Check sheet for the modelled part. Datum: model origin and axes. Units: mm. Round coordinates to 2 decimals unless told otherwise and drop trailing zeros. Order: outer loops, then holes, each group sorted by start corner. A loop starts at its lowest first (then second) coordinate and runs counter-clockwise, first axis right, second up.
(1) Thickness scan on probe 1 along Y at (x, z) = (24, 1.5); probe 2 along Y at (x, z) = (58, 4.25); probe 3 along Y at (x, z) = (66, 7.5). Record the ranges inside material, lowest first.
(2) Sectioned sample at A-A, the plane x = 42.5. Enter the section's corners in (y, z).
(3) Sectioned sample at C-C, the plane y = 44.5. Enter the section's corners in (x, z).
(4) Sectioned sample at D-D, the plane z = 4.75. Count the separate pieces of the cut face and the enclosed holes in it, and give its area (3 significant figures).
(5) Sectioned sample at B-B, the plane x = 117.5. Enter the section's corners in (y, z), and give its area (3 significant figures).
(6) Depth check by flat-ended pin: pin 1 (1 mm diameter, centred on y = 67.5, z = 3, fed in from -X); pin 2 (3 mm diameter, centred on y = 35, z = 4.5, fed in from -X); pin 3 (2 mm diameter, centred on x = 8.5, z = 5, fed in from +Y). Enter the tip coordinate at first touch or a pass-through.
```python
from build123d import *

# Parameters (mm, degrees)
F1_DEPTH = 8
F2_R     = 5


with BuildPart() as f1:
    # F0 (on Top) → F1 (new body)
    with BuildSketch(Plane.XY):
        with BuildLine():
            ThreePointArc((14.248786, 71.37788), (12.750499, 70.853022), (11.178073, 70.634359))
            ThreePointArc((11.178073, 70.634359), (8.837059, 69.762961), (7.469486, 67.672644))
            Line((7.469486, 67.672644), (-9.431398, 4.597688))
            ThreePointArc((-9.431398, 4.597688), (-9.031796, 1.562412), (-6.602971, -0.301292))
            Line((-6.602971, -0.301292), (-2.44949, -1.414214))
            ThreePointArc((-2.44949, -1.414214), (0.273796, -1.176889), (2.208717, 0.754093))
            ThreePointArc((2.208717, 0.754093), (2.633248, 1.34737), (3.242311, 1.748924))
            Line((3.242311, 1.748924), (4.121107, 2.119931))
            ThreePointArc((4.121107, 2.119931), (5.282511, 2.240283), (6.313193, 1.691615))
            ThreePointArc((6.313193, 1.691615), (8.106344, 0.656339), (10.176896, 0.656339))
            Line((10.176896, 0.656339), (73.564489, 17.640993))
            Line((73.564489, 17.640993), (99.557932, 24.605915))
            ThreePointArc((99.557932, 24.605915), (102.325731, 24.848066), (105.009431, 24.128971))
            Line((105.009431, 24.128971), (158.828727, -0.967379))
            ThreePointArc((158.828727, -0.967379), (161.88728, -1.100918), (164.144431, 0.967379))
            Line((164.144431, 0.967379), (165.96169, 4.864503))
            ThreePointArc((165.96169, 4.864503), (166.095229, 7.923056), (164.026931, 10.180207))
            Line((164.026931, 10.180207), (24.101743, 75.428393))
            ThreePointArc((24.101743, 75.428393), (21.621409, 75.724402), (19.449104, 74.491205))
            ThreePointArc((19.449104, 74.491205), (18.270863, 73.42721), (16.905718, 72.616827))
            Line((16.905718, 72.616827), (14.248786, 71.37788))
        make_face()
        with BuildLine():
            ThreePointArc((9.659258, 2.58819), (8.14162, 2.787991), (7.209769, 4.002404))
            Line((7.209769, 4.002404), (6.096847, 8.155885))
            ThreePointArc((6.096847, 8.155885), (6.296647, 9.673523), (7.51106, 10.605375))
            Line((7.51106, 10.605375), (70.586017, 27.506258))
            ThreePointArc((70.586017, 27.506258), (72.103655, 27.306458), (73.035506, 26.092045))
            Line((73.035506, 26.092045), (74.148428, 21.938564))
            ThreePointArc((74.148428, 21.938564), (73.948627, 20.420926), (72.734215, 19.489074))
            Line((72.734215, 19.489074), (9.659258, 2.58819))
        make_face(mode=Mode.SUBTRACT)
        with BuildLine():
            Line((17.418522, 65.006808), (0.517638, 1.931852))
            ThreePointArc((0.517638, 1.931852), (-0.414214, 0.717439), (-1.931852, 0.517638))
            Line((-1.931852, 0.517638), (-6.085333, 1.63056))
            ThreePointArc((-6.085333, 1.63056), (-7.299745, 2.562412), (-7.499546, 4.08005))
            Line((-7.499546, 4.08005), (9.401337, 67.155006))
            ThreePointArc((9.401337, 67.155006), (10.333189, 68.369419), (11.850827, 68.56922))
            Line((11.850827, 68.56922), (16.004308, 67.456298))
            ThreePointArc((16.004308, 67.456298), (17.218721, 66.524446), (17.418522, 65.006808))
        make_face(mode=Mode.SUBTRACT)
        with BuildLine():
            Line((158.711227, 8.245449), (156.893969, 4.348325))
            ThreePointArc((156.893969, 4.348325), (155.765393, 3.314176), (154.236117, 3.380946))
            Line((154.236117, 3.380946), (131.08432, 14.176806))
            ThreePointArc((131.08432, 14.176806), (130.050171, 15.305382), (130.116941, 16.834658))
            Line((130.116941, 16.834658), (131.934199, 20.731782))
            ThreePointArc((131.934199, 20.731782), (133.062775, 21.765931), (134.592051, 21.699161))
            Line((134.592051, 21.699161), (157.743848, 10.903301))
            ThreePointArc((157.743848, 10.903301), (158.777997, 9.774725), (158.711227, 8.245449))
        make_face(mode=Mode.SUBTRACT)
        with BuildLine():
            Line((81.875835, 24.009116), (80.762913, 28.162597))
            ThreePointArc((80.762913, 28.162597), (80.962714, 29.680235), (82.177127, 30.612087))
            Line((82.177127, 30.612087), (86.330608, 31.725009))
            ThreePointArc((86.330608, 31.725009), (87.848246, 31.525208), (88.780097, 30.310795))
            Line((88.780097, 30.310795), (89.893019, 26.157314))
            ThreePointArc((89.893019, 26.157314), (89.693218, 24.639676), (88.478806, 23.707825))
            Line((88.478806, 23.707825), (84.325325, 22.594903))
            ThreePointArc((84.325325, 22.594903), (82.807687, 22.794703), (81.875835, 24.009116))
        make_face(mode=Mode.SUBTRACT)
        with BuildLine():
            Line((96.089451, 32.701938), (97.906709, 36.599061))
            ThreePointArc((97.906709, 36.599061), (99.035284, 37.63321), (100.564561, 37.56644))
            Line((100.564561, 37.56644), (123.716358, 26.77058))
            ThreePointArc((123.716358, 26.77058), (124.750507, 25.642005), (124.683737, 24.112728))
            Line((124.683737, 24.112728), (122.866479, 20.215604))
            ThreePointArc((122.866479, 20.215604), (121.737903, 19.181456), (120.208626, 19.248225))
            Line((120.208626, 19.248225), (97.05683, 30.044086))
            ThreePointArc((97.05683, 30.044086), (96.022681, 31.172661), (96.089451, 32.701938))
        make_face(mode=Mode.SUBTRACT)
        with BuildLine():
            ThreePointArc((6.573737, 12.94241), (5.966531, 13.408336), (5.86663, 14.167155))
            Line((5.86663, 14.167155), (19.251114, 64.118731))
            Line((19.251114, 64.118731), (81.961415, 34.876437))
            ThreePointArc((81.961415, 34.876437), (82.478489, 34.31215), (82.445104, 33.547511))
            Line((82.445104, 33.547511), (82.416626, 33.48644))
            ThreePointArc((82.416626, 33.48644), (81.889586, 32.799588), (81.121649, 32.399825))
            Line((81.121649, 32.399825), (7.798482, 12.752942))
            ThreePointArc((7.798482, 12.752942), (7.539663, 12.718867), (7.280844, 12.752942))
            Line((7.280844, 12.752942), (6.573737, 12.94241))
        make_face(mode=Mode.SUBTRACT)
        with BuildLine():
            ThreePointArc((26.999238, 62.712477), (25.965089, 63.841052), (26.031859, 65.370329))
            Line((26.031859, 65.370329), (27.849117, 69.267453))
            ThreePointArc((27.849117, 69.267453), (28.977692, 70.301601), (30.506969, 70.234832))
            Line((30.506969, 70.234832), (89.688868, 42.637859))
            ThreePointArc((89.688868, 42.637859), (90.723016, 41.509284), (90.656247, 39.980007))
            Line((90.656247, 39.980007), (88.838988, 36.082884))
            ThreePointArc((88.838988, 36.082884), (87.710413, 35.048735), (86.181136, 35.115505))
            Line((86.181136, 35.115505), (26.999238, 62.712477))
        make_face(mode=Mode.SUBTRACT)
    extrude(amount=F1_DEPTH)

    # F2
    f2_edges = [f1.edges().sort_by_distance(p)[0] for p in [
        (19.251114, 64.118731, 4),
    ]]
    fillet(f2_edges, radius=F2_R)


solid = f1.part
```
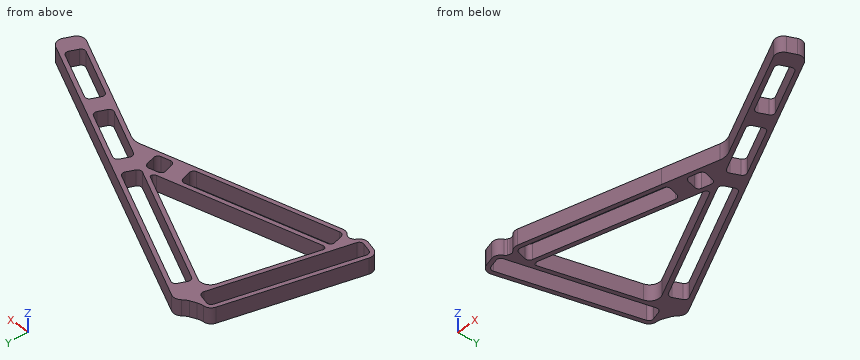
Derived:
1. probe 1: y = 4.36 to 6.43, 15.02 to 17.09, 61.85 to 75.47
1. probe 2: y = 13.47 to 15.54, 24.13 to 26.2, 46.05 to 48.26, 57.41 to 59.62
1. probe 3: y = 15.61 to 17.68, 26.28 to 28.35, 42.32 to 44.53, 53.68 to 55.89
2. outline: (9.32, 0) - (11.39, 0) - (11.39, 8) - (9.32, 8) - close; (19.98, 0) - (22.05, 0) - (22.05, 8) - (19.98, 8) - close; (53.28, 0) - (55.48, 0) - (55.48, 8) - (53.28, 8) - close; (64.64, 0) - (66.85, 0) - (66.85, 8) - (64.64, 8) - close
3. outline: (1.26, 0) - (3.33, 0) - (3.33, 8) - (1.26, 8) - close; (11.92, 0) - (13.99, 0) - (13.99, 8) - (11.92, 8) - close; (61.32, 0) - (66.06, 0) - (66.06, 8) - (61.32, 8) - close; (85.7, 0) - (90.43, 0) - (90.43, 8) - (85.7, 8) - close
4. separate pieces: 1
4. enclosed holes: 7
4. area: 1,760 mm2
5. outline: (18.3, 0) - (20.51, 0) - (20.51, 8) - (18.3, 8) - close; (29.67, 0) - (31.88, 0) - (31.88, 8) - (29.67, 8) - close
5. area: 35.3 mm2
6. pin 1: stops at x = 7.29
6. pin 2: stops at x = -1.69
6. pin 3: stops at y = 70.19
